Geometry: final body of the model. Coordinates: model frame, mm. Face numbers are marked on the shaded views. A direction names the side the tool comes from. Give positions to 0.01 mm unless a question says otherwise; leave off trailing zeros. Write each loop counter-clockwise with the first axis right and the second up, starting at its lowest first coordinate (ties: lowest second). Pieces come first, ordered by that corner, then holes. Notation, with made-up numbers: (45.25, 31.25) -> (101.25, 31.25) arc R20 cw to (101.25, 62.25) -> close; hole circle Ø2 at (39, -17). An arc over 180 degrees is marked (long way). Answer as a JSON object with one key per item and string values.
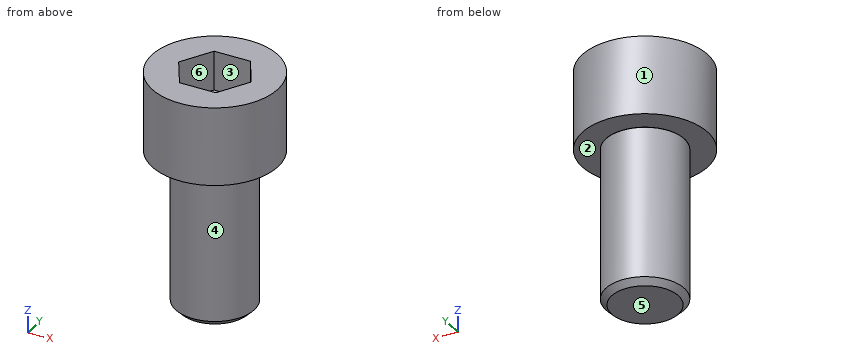
Solid Edge part; units mm, degrees
sketch "Sketch1" plane through (0, 0, 0) normal (0, 0, 1) x (1, 0, 0)
  circle A0 centre (0, 0) radius 8
extrude "Protrusion1" add sketch "Sketch1" along normal blind 10
sketch "Sketch2" plane through (0, 0, 0) normal (0, 0, -1) x (1, 0, 0)
  circle A0 centre (0, 0) radius 5
extrude "Protrusion2" add sketch "Sketch2" along normal blind 20
sketch "Sketch3" plane through (0, 0, -20) normal (0, 0, -1) x (1, 0, 0)
  circle A0 centre (0, 0) radius 4.9997
extrude "Cutout1" cut sketch "Sketch3" against normal blind 19.98 flip side to cut
chamfer "Chamfer_1" distance 0.75 angle 45 1 edges at (-4.9997, 0, -20)
sketch "Sketch4" plane through (0, 0, 10) normal (0, 0, 1) x (1, 0, 0)
  line L0 (-2.3094, 4) -> (2.3094, 4)
  line L1 (4.6188, 0) -> (2.3094, 4)
  line L2 (2.3094, -4) -> (4.6188, 0)
  line L3 (-2.3094, -4) -> (2.3094, -4)
  line L4 (-4.6188, 0) -> (-2.3094, -4)
  line L5 (-2.3094, 4) -> (-4.6188, 0)
extrude "Cutout2" cut sketch "Sketch4" against normal blind 5
properties part number "24104591"
Q1. Mould query, pull axis Y, two halves, no side actions, for the marked faces 1, 2 and 3. Classes: pulls with the +Y half, pulls with the -Y half, needs draft (parallel to the pull), parting line crosses it, or undercut.
Values:
{"face 1": "parting line crosses it", "face 2": "needs draft", "face 3": "undercut"}
Q2. Cut plane A-A (z = 6.25). Return the cut outline in (x, y).
Values:
{"outline": "circle Ø16 at (0, 0); hole (-4.62, 0) -> (-2.31, -4) -> (2.31, -4) -> (4.62, 0) -> (2.31, 4) -> (-2.31, 4) -> close"}
Q3. Cut plane C-C (z = -4). Return the cut outline in (x, y).
Values:
{"outline": "circle Ø10 at (0, 0)"}
Q4. Material intervals for L1, parallel to Z at x = 1, y = 0; L2, parallel to Z at x = 3.5, y = 5; L3, parallel to X at y = 6.25, z = 6.25, sorted ascending. Write a range as from..to.
Values:
{"L1": "-20..5", "L2": "0..10", "L3": "-4.99..4.99"}
Q5. First-contact query: P1, Ø6, axis at x = -3, z = -4.5, coming from the +Y side; P2, Ø2.5, axis at x = -1, z = 6.5, coming from the -Y side; P3, Ø4, axis at x = -0.5, y = -0.5, coming from the +Z side; P4, Ø2, axis at y = -2.5, z = 2, coming from the +X side. Flat tips, straight axial feed; report the tip coordinate or a pass-through.
Values:
{"P1": "y = 5", "P2": "y = -8", "P3": "z = 5", "P4": "x = 7.86"}
Q6. Cut plane D-D (x = -5.5). Return the cut outline in (y, z).
Values:
{"outline": "(-5.81, 0) -> (5.81, 0) -> (5.81, 10) -> (-5.81, 10) -> close"}
Q7. Set-up query: the marked faces 4, 5 and 6. Return all of +Z, -Z, +X, -X, +Y, -Y with unobstructed straight access to the full face (end or side cutting, diameter ignored); none if empty.
Values:
{"face 4": "-Z", "face 5": "-Z, +X, -X, +Y, -Y", "face 6": "+Z"}
